```python
from build123d import *

# Parameters (mm, degrees)
SKETCH1_W           = 8.49
SKETCH1_H           = 10.5
SKETCH1_W_2         = 9.29
SKETCH1_H_2         = 2
BOSS_EXTRUDE1_DEPTH = 2.3


with BuildPart() as part:
    # Sketch1 → Boss-Extrude1 (new body)
    with BuildSketch(Plane.XY):
        Polygon((0, 0), (0, -2), (2.5, -2), (2.5, 0), (10.99, 0), (10.99, -2), (13.49, -2), (13.49, 0), (13.49, 18), (0, 18), align=None)
        with Locations((6.745, 7.75)):
            Rectangle(SKETCH1_W, SKETCH1_H, mode=Mode.SUBTRACT)
        with Locations((6.745, 15.5)):
            Rectangle(SKETCH1_W_2, SKETCH1_H_2, mode=Mode.SUBTRACT)
    extrude(amount=BOSS_EXTRUDE1_DEPTH)


solid = part.part
```
Could you check a few things on this model? Use its own coordinates, in mm. A direction names the side the tool comes from. Give positions to 0.01 mm unless a question says otherwise; leave off trailing zeros. Write each loop counter-clockwise with the first axis right and the second up, starting at its lowest first coordinate (ties: lowest second). Pieces come first, ordered by that corner, then holes. Notation, with made-up numbers: (-9, 83) - (35, 83) arc R15 cw to (35, 103) - close; hole circle Ø3 at (34.25, -2). An arc over 180 degrees is marked (long way). One line per item, written item: value. Start each with the question number.
Item 1: If we mould it in two halves opening along X, with no side actions, what happens to faces 4 (the face through (2, 8, 2.3)), 5 (the face through (13.49, 8, 1)), 6 (the face through (7, 16.5, 1))? For each: +X half, -X half, draft (parallel to the pull), parting line (faces both ways), or undercut.
Item 2: Which directions (+Z, -Z, +X, -X, +Y, -Y) give clear straight access to the entire face, cutting with the end or side of a thin tool? Please do faces 1 (the face through (12, -2, 1)), 2 (the face through (11.39, 15, 1)), 3 (the face through (2.5, -1, 1)).
Item 3: Please list where these lines run through material, in increasing order: line 1 (Y direction, x = 5.5, z = 0.25); line 2 (X direction, y = -0.75, z = 0.9); line 3 (X direction, y = 15.75, z = 2). Write a range as from..to.
Item 4: Imagine slicing it at C-C, the plane x = 9.25. List the corners of the cut face in (y, z) for me.
Item 5: I'm going to push a flat-ended pin straight in: pin 1 (0.7 mm diameter, centred on x = 5, z = 1, fed in from -Y). Where does the tip first touch, or does it pass through?
Item 6: Imagine slicing it at D-D, the plane y = 11.5. List the corners of the cut face in (x, z) for me, and give its area (3 significant figures).
Item 7: Imagine slicing it at A-A, the plane y = 15.25. List the corners of the cut face in (x, z) for me, and give its area (3 significant figures).
Item 8: Imagine slicing it at B-B, the plane z = 0.25. List the corners of the cut face in (x, y) for me, and give its area (3 significant figures).
Geometry says:
1. face 4: draft
1. face 5: +X half
1. face 6: undercut
2. face 1: +Z, -Z, +X, -X, -Y
2. face 2: +Z, -Z
2. face 3: +Z, -Z, -Y
3. line 1: 0..2.5, 13..14.5, 16.5..18
3. line 2: 0..2.5, 10.99..13.49
3. line 3: 0..2.1, 11.39..13.49
4. outline: (0, 0) - (2.5, 0) - (2.5, 2.3) - (0, 2.3) - close; (13, 0) - (14.5, 0) - (14.5, 2.3) - (13, 2.3) - close; (16.5, 0) - (18, 0) - (18, 2.3) - (16.5, 2.3) - close
5. pin 1: y = 0
6. outline: (0, 0) - (2.5, 0) - (2.5, 2.3) - (0, 2.3) - close; (10.99, 0) - (13.49, 0) - (13.49, 2.3) - (10.99, 2.3) - close
6. area: 11.5 mm^2
7. outline: (0, 0) - (2.1, 0) - (2.1, 2.3) - (0, 2.3) - close; (11.39, 0) - (13.49, 0) - (13.49, 2.3) - (11.39, 2.3) - close
7. area: 9.66 mm^2
8. outline: (0, -2) - (2.5, -2) - (2.5, 0) - (10.99, 0) - (10.99, -2) - (13.49, -2) - (13.49, 18) - (0, 18) - close; hole (2.1, 14.5) - (11.39, 14.5) - (11.39, 16.5) - (2.1, 16.5) - close; hole (2.5, 2.5) - (10.99, 2.5) - (10.99, 13) - (2.5, 13) - close
8. area: 145 mm^2
